Could you check a few things on this model? Use its own coordinates, in mm. A direction names the side the tool comes from. Round coordinates to 2 decimals unless told otherwise and drop trailing zeros. One line per question, with ' | ' between items. Start each with the question number.
1. For faces 1 (the flat face through (-9, -9, 25)), 2 (the flat face through (-27, -4.959, 12)), 3 (the flat face through (-19, -17, 22.494)), 4 (the cylindrical face through (-21.006, -20.571, 2.256)), 5 (the flat face through (4.959, -26, 12)), which set-ups out of +Z, -Z, +X, -X, +Y, -Y let a thin tool reach every point of the face, with its end or its side?
2. Thinking about a two-plate mould opening in X: for faces 6 (the flat face through (-27, 4.959, 12)), 7 (the flat face through (0, -9.48, 12)), 8 (the cylindrical face through (-42.8, -8, 12.3)), 9 (the flat face through (-4.959, -27, 12)), which applies, released by +X, released by -X, zero draft, split by the parting line, or undercut?
3. If I drill on line 1 along X through (y, z) = (-14, 2.5); line 2 along X through (y, z) = (4, 8.75); line 3 along Z through (x, y) = (-23, -16), over which ranges is the centre line in solid material (lowest first)? Write a range as [from, to].
4. For pin 1 Ø3 at (y, z) = (-9.5, 17.5) entering from +X; pin 2 Ø1.5 at (x, z) = (-13.5, 3.5) entering from -Y; pin 3 Ø10 at (y, z) = (-29, 9.5) entering from -X; pin 4 Ø15 at (x, y) = (-24.5, -28.5) entering from -Z, each with a flat end and sliding along its axis, tell me the tip position at first contact or that it passes through.
from build123d import *

# Parameters (mm, degrees)
F1_DEPTH    = 25
F2_W        = 30.2227726206
F2_H        = 20.068306243
F3_DEPTH    = 34
F4_T1_DEPTH = 45.2364697276
F5_R        = 5


# Not quite as in the source:
# - a fillet or chamfer that OpenCascade refuses, or shapes differently, is made with other operations: its cross-section is extruded or revolved along the edge and cut away or added


with BuildPart() as f1:
    # F0 (on Top) → F1 (new body)
    with BuildSketch(Plane.XY):
        with BuildLine():
            Line((-4.959, -9.4801727682), (4.959, -9.4801727682))
            Line((4.959, -9.4801727682), (4.959, -43.3722550981))
            Line((4.959, -43.3722550981), (8.959, -43.3722550981))
            add(Edge.make_bspline(
                [(8.959, -43.3722550981), (10.9444993843, -36.8281108572), (14.7331593025, -24.340805557), (6.9032731799, -9.0055840914), (9.6423102918, 4.2067701187), (11.0949236172, 11.2137733098)],
                knots=[0, 0, 0, 0, 0.3408719694, 0.6504398731, 1, 1, 1, 1], degree=3))
            add(Edge.make_bspline(
                [(-43.8664413989, 8.959), (-38.2964370805, 10.3608151634), (-26.1129886059, 13.4270502754), (-0.196589781, 7.3008338793), (7.8789436209, 10.0993137603), (11.0949236172, 11.2137733098)],
                knots=[0, 0, 0, 0, 0.3363503338, 0.7357098355, 1, 1, 1, 1], degree=3))
            Line((-43.8664413989, 8.959), (-43.8664413989, 4.959))
            Line((-43.8664413989, 4.959), (-10, 4.959))
            Line((-10, 4.959), (-10, -4.959))
            Line((-10, -4.959), (-43.8664413989, -4.959))
            Line((-43.8664413989, -4.959), (-43.8664413989, -8.959))
            ThreePointArc((-43.8664413989, -8.959), (-22.3244394728, -19.3298404084), (-9.7910396518, -39.6897536373))
            ThreePointArc((-9.7910396518, -39.6897536373), (-8.0019231601, -42.3463897646), (-4.9677422736, -43.3722550981))
            Line((-4.9677422736, -43.3722550981), (-4.959, -43.3722550981))
            Line((-4.959, -43.3722550981), (-4.959, -9.4801727682))
        make_face()
    extrude(amount=F1_DEPTH)

    # F2 (on face) → F3 (cut)
    with BuildSketch(Plane(origin=(-43.8664413989, 0, 0), x_dir=(0, -1, 0), z_dir=(-1, 0, 0))):
        with Locations((24.5702010579, 12.4597531976)):
            Rectangle(F2_W, F2_H)
    extrude(amount=-F3_DEPTH, mode=Mode.SUBTRACT)

    # F4: fillet of radius 5 on 1 edges, made by hand

    # F4_s2 → F4_t1 (cut)
    with BuildSketch(Plane.XY.offset(-10.1182348638)):
        with BuildLine():
            ThreePointArc((-40.1210831358, -9.7517343717), (-42.8207560477, -7.971672665), (-43.8664413989, -4.9117060545))
            Line((-43.8664413989, -4.9117060545), (-43.8664413989, -8.959))
            ThreePointArc((-43.8664413989, -8.959), (-41.9848306621, -9.3131688624), (-40.1210831358, -9.7517343717))
        make_face()
    extrude(amount=F4_T1_DEPTH, mode=Mode.SUBTRACT)

    # F5
    f5_edges = [f1.edges().sort_by_distance(p)[0] for p in [
        (8.959, -43.372255, 12.5),
        (11.094924, 11.213773, 12.5),
        (-43.866441, 8.959, 12.5),
    ]]
    fillet(f5_edges, radius=F5_R)


solid = f1.part
Geometry results:
1) face 1: +Z, +X, -X, +Y, -Y | face 2: +Z, -Z, -X | face 3: -X, -Y | face 4: +Z, -Z, -X, -Y | face 5: +Z, -Z, -Y
2) face 6: zero draft | face 7: undercut | face 8: released by -X | face 9: undercut
3) line 1: x = [-9.87, -4.96], [4.96, 10.03] | line 2: x = [-10, 9.66] | line 3: z = [0, 2.43], [22.49, 25]
4) pin 1: stops at x = 9.3 | pin 2: stops at y = -9.46 | pin 3: stops at x = -9.87 | pin 4: passes through
